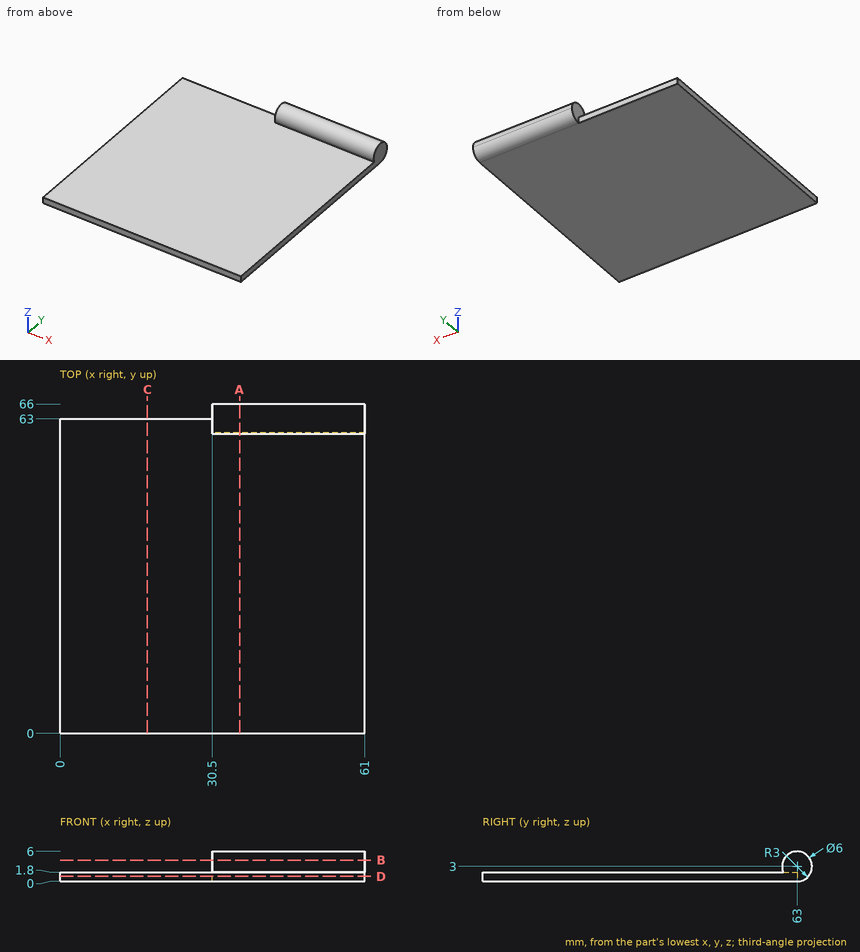
Geometry check sheet. Reference: drawing and pictorial views, mm from the part's lowest x, y, z. Coordinates: 2 decimals unless noted, no trailing zeros. Loops run counter-clockwise (first coordinate to the right, second up) from the corner with the lowest first, then second, coordinate; pieces in that order, holes last. Notation, with made-up numbers: (21.5, -22) -> (43.5, -22) arc R17 cw to (43.5, -16) -> close; hole circle Ø4 at (-32.5, 64.25). An arc over 180 degrees is marked (long way). Write item = value, one per line. Start each with the question number.
1. Material ranges on line 1 (Z direction, x = 37.5, y = 58); line 2 (Y direction, x = 8, z = 1); line 3 (Y direction, x = 56, z = 5.75), recorded low to high.
2. Section check B-B on z = 4.25. Record the cut outline in (x, y), then the cut area to 3 significant figures.
3. Section check C-C on x = 17.5. Record the cut outline in (y, z), then the cut area to 3 significant figures.
4. Depth check by flat-ended pin: P1, Ø2, axis at x = 34, y = 31.5, coming from the +Z side; P2, Ø3, axis at y = 62.5, z = 3, coming from the -X side; P3, Ø0.9, axis at x = 20.5, z = 1, coming from the +Y side. Enter the tip coordinate at first touch or a pass-through.
5. Section check A-A on x = 36. Record the cut outline in (y, z).
6. Section check D-D on z = 1. Record the cut outline in (x, y), then the cut area to 3 significant figures.
Responses:
q1.line_1 = 0 to 1.8
q1.line_2 = 0 to 63
q1.line_3 = 61.8 to 64.2
q2.outline = (30.5, 60.27) -> (61, 60.27) -> (61, 65.73) -> (30.5, 65.73) -> close
q2.area = 166 mm2
q3.outline = (0, 0) -> (63, 0) -> (63, 1.8) -> (0, 1.8) -> close
q3.area = 113 mm2
q4.P1 = 1.8
q4.P2 = 0
q4.P3 = 63
q5.outline = (0, 0) -> (63, 0) arc R3 ccw (long way) to (60.25, 1.8) -> (0, 1.8) -> close
q6.outline = (0, 0) -> (61, 0) -> (61, 65.24) -> (30.5, 65.24) -> (30.5, 63) -> (0, 63) -> close
q6.area = 3,910 mm2
